Here's how the part is built. I have some questions about the finished solid (model axes, mm). Give positions to 0.01 mm unless a question says otherwise; leave off trailing zeros. Write each loop counter-clockwise with the first axis right and the second up, starting at its lowest first coordinate (ties: lowest second). Pieces come first, ordered by that corner, then holes. Notation, with made-up numbers: M 87.5,21 L 99.5,21 A13 ccw 99.5,46 Z; hole C -23.75,38.5 d10. An arc over 180 degrees is marked long. Use one line per item in the form item = value. Start each with the question number.
from build123d import *

# Parameters (mm, degrees)
SKETCH_1_W          = 40
SKETCH_1_H          = 40
EXTRUDE_1_DEPTH     = 40
CUT_EXTRUDE_1_DEPTH = 77.035731628
CUT_EXTRUDE_2_DEPTH = 62.629021291


with BuildPart() as part:
    # Эскиз1 → Бобышка-Вытянуть1 (new body)
    with BuildSketch(Plane(origin=(0, 0, 0), x_dir=(1, 0, 0), z_dir=(0, 1, 0))):
        with Locations((-30.807799443, -4.456824513)):
            Rectangle(SKETCH_1_W, SKETCH_1_H)
    extrude(amount=EXTRUDE_1_DEPTH)

    # Эскиз2 → Вырез-Вытянуть1 (cut, through all)
    with BuildSketch(Plane(origin=(0, 0, -15.543175487), x_dir=(-1, 0, 0), z_dir=(0, 0, -1))):
        Polygon((10.807799443, 40), (10.807799443, 0), (20.807799443, 0), align=None)
    extrude(amount=-CUT_EXTRUDE_1_DEPTH, mode=Mode.SUBTRACT)

    # Эскиз3 → Вырез-Вытянуть2 (cut, through all)
    with BuildSketch(Plane.ZY.offset(50.807799443)):
        Polygon((24.456824513, 0), (14.456824513, 0), (24.456824513, 40), align=None)
    extrude(amount=-CUT_EXTRUDE_2_DEPTH, mode=Mode.SUBTRACT)


solid = part.part
1) Will these pins go through, and if not, where does the flat tip stop? P1, Ø5, axis at y = 5.5, z = 0, coming from the +X side; P2, Ø10, axis at y = 17.5, z = -3, coming from the +X side; P3, Ø1.5, axis at y = 16, z = -5.5, coming from the +X side.
2) Please list where these lines run through material, in increasing order: line 1 (X direction, y = 29.5, z = 7.5); line 2 (Z direction, x = -43, y = 34.5); line 3 (X direction, y = 31.5, z = 8).
3) Suppose I cut it at A-A, the plane x = -25. List the corners of the cut face in (y, z) for me, and give its area (3 significant figures).
4) Suppose I cut it at B-B, the plane z = -6.5. List the corners of the cut face in (x, y) for me, and give its area (3 significant figures).
5) Thinking about a two-plate mould opening in X: for faces 1 (the face through (-50.808, 20, 0)), 2 (the face through (-36, 0, -1)), 3 (the face through (-15.878, 19.72, -0.268)), which applies, released by +X, released by -X, zero draft, split by the parting line, or undercut?
Checks:
q1.P1 = -18.81
q1.P2 = -15.18
q1.P3 = -16.62
q2.line_1 = -50.81 to -13.43
q2.line_2 = -15.54 to 23.08
q2.line_3 = -50.81 to -12.93
q3.outline = M 0,-15.54 L 40,-15.54 L 40,24.46 L 0,14.46 Z
q3.area = 1,400 mm^2
q4.outline = M -50.81,0 L -20.81,0 L -10.81,40 L -50.81,40 Z
q4.area = 1,400 mm^2
q5.face_1 = released by -X
q5.face_2 = zero draft
q5.face_3 = released by +X
